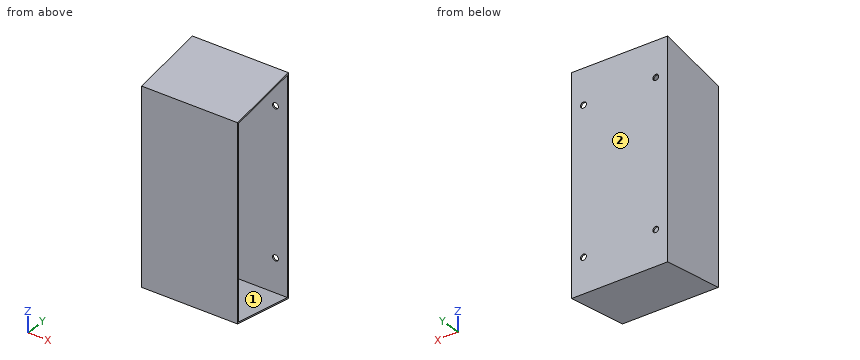
from build123d import *

# Parameters (mm, degrees)
BOSS_EXTRUDE1_DEPTH = 3.175
BOSS_EXTRUDE2_DEPTH = 203.2
SKETCH3_R           = 6.35
CUT_EXTRUDE1_DEPTH  = 3.175


with BuildPart() as part:
    # Sketch1 → Boss-Extrude1 (new body)
    with BuildSketch(Plane(origin=(0, 0, 0), x_dir=(0, 0, -1), z_dir=(1, 0, 0))):
        Polygon((-358.316862416, 16.748657718), (-383.716862416, 169.148657718), (83.008137584, 169.148657718), (57.608137584, 16.748657718), align=None)
    extrude(amount=BOSS_EXTRUDE1_DEPTH)

    # Sketch2 → Boss-Extrude2 (add)
    with BuildSketch(Plane(origin=(3.175, 0, 0), x_dir=(0, 0, -1), z_dir=(1, 0, 0))):
        Polygon((-383.716862416, 169.148657718), (-358.316862416, 16.748657718), (57.608137584, 16.748657718), (83.008137584, 169.148657718), align=None)
        Polygon((54.918509078, 19.923657718), (79.260175745, 165.973657718), (-379.968900577, 165.973657718), (-355.62723391, 19.923657718), align=None, mode=Mode.SUBTRACT)
    extrude(amount=BOSS_EXTRUDE2_DEPTH)

    # Sketch3 → Cut-Extrude1 (cut)
    with BuildSketch(Plane(origin=(0, 169.148657718, 0), x_dir=(1, 0, 0), z_dir=(0, 1, 0))):
        with Locations((180.975, 6.808137584)):
            Circle(SKETCH3_R)
        with Locations((25.4, 6.808137584)):
            Circle(SKETCH3_R)
        with Locations((25.4, -307.516862416)):
            Circle(SKETCH3_R)
        with Locations((180.975, -307.516862416)):
            Circle(SKETCH3_R)
    extrude(amount=-CUT_EXTRUDE1_DEPTH, mode=Mode.SUBTRACT)


solid = part.part
Here's how the part is built. I have some questions about the finished solid (model axes, mm). Face numbers are marked on the shaded views. A direction names the side the tool comes from. Round coordinates to 2 decimals unless told otherwise and drop trailing zeros. Write each loop counter-clockwise with the first axis right and the second up, starting at its lowest first coordinate (ties: lowest second). Pieces come first, ordered by that corner, then holes. Notation, with made-up numbers: (4, 38) -> (57, 38) arc R19 ccw to (57, 72) -> close; hole circle Ø10 at (84, 8.5). An arc over 180 degrees is marked (long way). One line per item, written item: value.
1) If I drill on line 1 (Y direction, x = 73, z = -51.5); line 2 (Z direction, x = 25.4, y = 167); line 3 (X direction, y = 52, z = 40) (3 decimals), over which ranges is the centre line in solid material (lowest first)? Write a range as [from, to].
Filled sheet:
line 1: y = [16.75, 19.92], [165.97, 169.15]
line 2: z = [-82.65, -13.16], [-0.46, 301.17], [313.87, 383.36]
line 3: x = [0, 3.175]
2) Suppose I cut it at B-B on x = 69. List the corners of the cut face in (y, z) for me, plus the area to 3 significant figures.
Filled sheet:
outline: (16.75, -57.61) -> (169.15, -83.01) -> (169.15, 383.72) -> (16.75, 358.32) -> close; hole (19.92, -54.92) -> (165.97, -79.26) -> (165.97, 379.97) -> (19.92, 355.63) -> close
area: 3,740 mm2
3) For the marked faces 1 and 2, which set-ups out of +Z, -Z, +X, -X, +Y, -Y let a thin tool reach every point of the face, with its end or its side?
Filled sheet:
face 1: +X
face 2: +Z, -Z, +X, -X, +Y
4) I'm going to push flat-ended pins straight in: pin 1 Ø6 at (y, z) = (92.5, 218.5) entering from -X; pin 2 Ø11.5 at (x, z) = (25.4, 307.52) entering from +Y; pin 3 Ø2 at (y, z) = (123.5, 250) entering from +X (3 decimals); pin 4 Ø3 at (x, y) = (50, 33.5) entering from +Z. Where does each tip first touch, or does it pass through?
Filled sheet:
pin 1: stops at x = 0
pin 2: stops at y = 19.92
pin 3: stops at x = 3.175
pin 4: stops at z = 361.36
5) Suppose I cut it at D-D on y = 80. List the corners of the cut face in (x, z) for me (3 decimals), plus the area to 3 significant figures.
Filled sheet:
outline: (0, -68.15) -> (206.375, -68.15) -> (206.375, -64.931) -> (3.175, -64.931) -> (3.175, 365.64) -> (206.375, 365.64) -> (206.375, 368.859) -> (0, 368.859) -> close
area: 2,700 mm2
6) Suppose I cut it at A-A on x = 25.4. List the corners of the cut face in (y, z) for me, plus the area to 3 significant figures.
Filled sheet:
outline: (16.75, -57.61) -> (169.15, -83.01) -> (169.15, -13.16) -> (165.97, -13.16) -> (165.97, -79.26) -> (19.92, -54.92) -> (19.92, 355.63) -> (165.97, 379.97) -> (165.97, 313.87) -> (169.15, 313.87) -> (169.15, 383.72) -> (16.75, 358.32) -> close; (165.97, -0.46) -> (169.15, -0.46) -> (169.15, 301.17) -> (165.97, 301.17) -> close
area: 3,660 mm2
7) Suppose I cut it at C-C on z = 265. List the corners of the cut face in (x, y) for me (3 decimals), plus the area to 3 significant figures.
Filled sheet:
outline: (0, 16.749) -> (206.375, 16.749) -> (206.375, 19.924) -> (3.175, 19.924) -> (3.175, 165.974) -> (206.375, 165.974) -> (206.375, 169.149) -> (0, 169.149) -> close
area: 1,770 mm2
